Input: part model. Units: mm. Frame: model coordinates. Face numbers are marked on the shaded views. A direction names the side the tool comes from. Give positions to 0.01 mm unless a question says otherwise; leave off trailing zeros. Write each loop counter-clockwise with the first axis right and the second up, starting at its lowest first coordinate (ties: lowest second). Pieces come first, ordered by that corner, then holes. Notation, with made-up numbers: (68.25, 87.5) - (124.25, 87.5) arc R27 ccw to (124.25, 117.5) - close; hole circle Ø3 at (20, 62.5). An arc over 180 degrees is marked (long way). Answer as a JSON object with one key per item and string values. Group by question number.
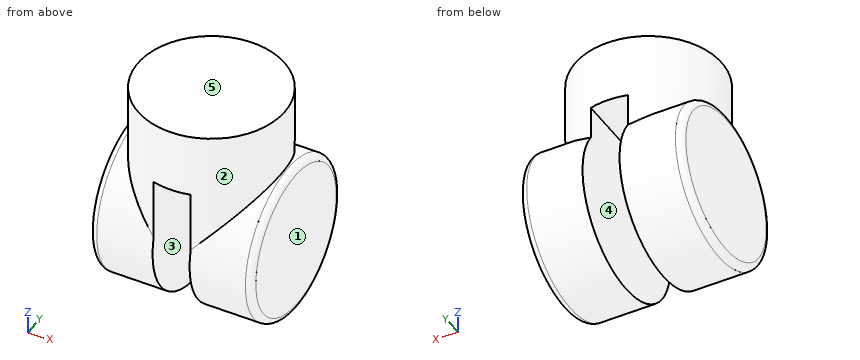
from build123d import *

# Parameters (mm, degrees)
SKETCH1_R               = 62.738
BOSS_EXTRUDE1_DEPTH     = 129.032
FILLET1_R               = 5.334
FILLET2_R               = 5.334
CUT_EXTRUDE1_DEPTH      = 157.593008583
CUT_EXTRUDE1_DEPTH_BACK = 157.593008583
SKETCH2_W               = 29.464
SKETCH2_H               = 125.476
BOSS_EXTRUDE2_START     = 10.518
BOSS_EXTRUDE2_OUTLINE_R = 58
BOSS_EXTRUDE2_DEPTH     = 103.032
CUT_EXTRUDE2_DEPTH      = 184.092449966
CUT_EXTRUDE2_DEPTH_BACK = 184.092449966
SKETCH3_W               = 29.464
SKETCH3_H               = 125.5


# Read off the part's stored shape, not the designer's step: Boss-Extrude2
with BuildPart() as part:
    # Sketch1 → Boss-Extrude1 (new body)
    with BuildSketch(Plane(origin=(0, 0, 0), x_dir=(0, 0, -1), z_dir=(1, 0, 0))):
        Circle(SKETCH1_R)
    extrude(amount=BOSS_EXTRUDE1_DEPTH)

    # Fillet1
    fillet1_edges = [part.edges().sort_by_distance(p)[0] for p in [
        (0, 0, 62.738),
    ]]
    fillet(fillet1_edges, radius=FILLET1_R)

    # Fillet2
    fillet2_edges = [part.edges().sort_by_distance(p)[0] for p in [
        (129.032, 0, 62.738),
    ]]
    fillet(fillet2_edges, radius=FILLET2_R)

    # Sketch2 → Cut-Extrude1 (cut, two sides: drawn at the far end of the back side and taken through both)
    with BuildSketch(Plane.XY.offset(-CUT_EXTRUDE1_DEPTH_BACK)):
        with Locations((64.516, 0)):
            Rectangle(SKETCH2_W, SKETCH2_H)
    extrude(amount=CUT_EXTRUDE1_DEPTH + CUT_EXTRUDE1_DEPTH_BACK, mode=Mode.SUBTRACT)


with BuildPart() as cut_extrude1_piece_1:
    # of the separate pieces the step leaves, piece 1, a body of its own (cut_extrude1_pieces)
    add(part.part.solids().sort_by_distance((5.334, 0, -62.738))[0])



with BuildPart() as cut_extrude1_piece_2:
    # of the separate pieces the step leaves, piece 2, a body of its own (cut_extrude1_pieces)
    add(part.part.solids().sort_by_distance((79.248, 0, -62.738))[0])


with BuildPart() as cut_extrude1_piece_1_1:
    add(cut_extrude1_piece_1.part)

    add(cut_extrude1_piece_2.part)  # Boss-Extrude2 merges Cut-Extrude1 piece 2
    # Boss-Extrude2 outline → Boss-Extrude2 (add)
    with BuildSketch(Plane.XY.offset(BOSS_EXTRUDE2_START)):
        with Locations((64.483080673, -5.087127651)):
            Circle(BOSS_EXTRUDE2_OUTLINE_R)
    extrude(amount=BOSS_EXTRUDE2_DEPTH)

    # Sketch3 → Cut-Extrude2 (cut, two sides: drawn at the far end of the back side and taken through both)
    with BuildSketch(Plane(origin=(0, 0, 0), x_dir=(1, 0, 0), z_dir=(0, 1, 0)).offset(-CUT_EXTRUDE2_DEPTH_BACK)):
        with Locations((64.516, -0.012)):
            Rectangle(SKETCH3_W, SKETCH3_H)
    extrude(amount=CUT_EXTRUDE2_DEPTH + CUT_EXTRUDE2_DEPTH_BACK, mode=Mode.SUBTRACT)


solid = cut_extrude1_piece_1_1.part
1) Reachability of the marked faces 4 and 5 from +Z, -Z, +X, -X, +Y, -Y: full face, straight path, thin tool, end or side. Return the list, or none.
2) Cut plane C-C on x = 20. Return the cut outline in (y, z).
3) Line query: line 1 along X through (y, z) = (44.5, 30); line 2 along Z through (x, y) = (66, 42.5); line 3 along X through (y, z) = (31, 51.5). Output: solid intervals per line, ascending. Write a range as from..to.
4) Pin query (flat end, axial travel): P1, Ø5, axis at y = -29, z = 72.5, coming from the +X side; P2, Ø1.5, axis at x = 23.5, z = 2, coming from the +Y side; P3, Ø14.5, axis at x = 71, y = -17.5, coming from the -Z side. Return the tip coordinate at first contact, or that it passes through.
5) Cut plane D-D on x = 108.5. Return the cut outline in (y, z).
6) Cut plane A-A on z = 0. Return the cut outline in (x, y).
7) Cut plane B-B on y = 0. Return the cut outline in (x, z).
8) Mould query, pull axis X, two halves, no side actions, for the marked faces 1, 2 and 3. Classes: +X half, -X half, draft (parallel to the pull), parting line (faces both ways), or undercut.
Filled in:
{
 "1": {"face 4": "-Z, +Y, -Y", "face 5": "+Z, +X, -X, +Y, -Y"},
 "2": {"outline": "(-42.31, 46.33) arc R62.74 ccw (long way) to (32.13, 53.89) - (32.13, 113.55) - (-42.31, 113.55) - close"},
 "3": {"line 1": "x = 0..49.78, 79.25..129.03", "line 2": "z = 62.76..113.55", "line 3": "x = 0.74..49.78, 79.25..128.29"},
 "4": {"P1": "stops at x = 118.39", "P2": "stops at y = 62.73", "P3": "stops at z = 62.76"},
 "5": {"outline": "(-42.86, 45.82) arc R62.74 ccw (long way) to (32.68, 53.55) - (32.68, 113.55) - (-42.86, 113.55) - close"},
 "6": {"outline": "(0, -57.4) arc R5.33 ccw to (5.33, -62.74) - (49.78, -62.74) - (49.78, 62.74) - (5.33, 62.74) arc R5.33 ccw to (0, 57.4) - close; (79.25, -62.74) - (123.7, -62.74) arc R5.33 ccw to (129.03, -57.4) - (129.03, 57.4) arc R5.33 ccw to (123.7, 62.74) - (79.25, 62.74) - close"},
 "7": {"outline": "(0, -57.4) arc R5.33 ccw to (5.33, -62.74) - (49.78, -62.74) - (49.78, 62.76) - (79.25, 62.76) - (79.25, -62.74) - (123.7, -62.74) arc R5.33 ccw to (129.03, -57.4) - (129.03, 57.4) arc R5.33 ccw to (123.7, 62.74) - (122.26, 62.74) - (122.26, 113.55) - (6.71, 113.55) - (6.71, 62.74) - (5.33, 62.74) arc R5.33 ccw to (0, 57.4) - close"},
 "8": {"face 1": "+X half", "face 2": "parting line", "face 3": "undercut"}
}
